Can you work these out from the model? Positions are in its coordinate system, mm. A direction names the side the tool comes from. Coordinates: 2 decimals unless noted, no trailing zeros. Write each loop counter-clockwise with the first axis right and the second up, starting at its lowest first coordinate (ties: lowest second). Pieces come first, ordered by that corner, then holes. Notation, with made-up numbers: (48, 61.5) -> (64, 61.5) arc R35 ccw to (64, 94.5) -> close; hole circle Ø11 at (61, -4). An arc over 180 degrees is marked (long way). Answer as CSV lines item,"result". Start each with the question number.
```python
from build123d import *

# Parameters (mm, degrees)
EXTRUDE_1_DEPTH            = 11.7
EXTRUDE_2_DEPTH            = 20
SKETCH_3_W                 = 3
SKETCH_3_H                 = 2.35
EXTRUDE_3_DEPTH            = 20
EXTRUDE_4_DEPTH            = 28.3
SKETCH_5_W                 = 2.35
SKETCH_5_H                 = 60
EXTRUDE_5_DEPTH            = 14.7
CUT_EXTRUDE_1_REACH        = 70.066
SKETCH_6_W                 = 11
SKETCH_6_H                 = 2.6
CUT_EXTRUDE_2_REACH        = 70.066
CUT_EXTRUDE_3_REACH        = 70.066
HOLE_WIZARD_3_0_3_1_D      = 3
HOLE_WIZARD_3_0_3_1_DEPTH  = 19.132814283
HOLE_WIZARD_3_0_3_2_D      = 3
HOLE_WIZARD_3_0_3_2_DEPTH  = 2.35
HOLE_WIZARD_15_0_15_1_D    = 15
HOLE_WIZARD_3_0_3_3_REACH  = 65.316
HOLE_WIZARD_3_0_3_3_BORE_R = 1.5
HOLE_WIZARD_3_0_3_4_REACH  = 68.474
HOLE_WIZARD_3_0_3_4_BORE_R = 1.5
FILLET_1_R                 = 1
FILLET_2_R                 = 2
FILLET_START               = 2.9999999
FILLET_3_DEPTH             = 3.0000001
FILLET_START_2             = -60
FILLET_3_2_DEPTH           = 60


with BuildPart() as part:
    # Эскиз1 → Бобышка-Вытянуть1 (new body)
    with BuildSketch(Plane(origin=(0, 0, 0), x_dir=(1, 0, 0), z_dir=(0, 1, 0))):
        with BuildLine():
            Line((9, 21.5), (6, 21.5))
            Line((6, 21.5), (6, 8.5))
            Line((6, 8.5), (-10.132814283, 8.5))
            Line((-10.132814283, 8.5), (-8.930469533, -1.11656344))
            ThreePointArc((-8.930469533, -1.11656344), (0.55936312, -8.982600564), (9, 0))
            Line((9, 0), (9, 21.5))
        make_face()
    extrude(amount=-EXTRUDE_1_DEPTH)

    # Эскиз2 → Бобышка-Вытянуть2 (add)
    with BuildSketch(Plane.XZ.offset(11.7)):
        with BuildLine():
            Line((9, -8.5), (-10.132814283, -8.5))
            Line((-10.132814283, -8.5), (-8.930469533, 1.11656344))
            ThreePointArc((-8.930469533, 1.11656344), (0.55936312, 8.982600564), (9, 0))
            Line((9, 0), (9, -8.5))
        make_face()
    extrude(amount=EXTRUDE_2_DEPTH)

    # Эскиз3 → Бобышка-Вытянуть3 (add)
    with BuildSketch(Plane.XZ.offset(11.7)):
        with Locations((7.5, -20.325)):
            Rectangle(SKETCH_3_W, SKETCH_3_H)
    extrude(amount=EXTRUDE_3_DEPTH)

    # Эскиз4 → Бобышка-Вытянуть4 (add)
    with BuildSketch(Plane.XZ.offset(31.7)):
        with BuildLine():
            Line((6, -21.5), (6, -8.5))
            Line((6, -8.5), (-10.132814283, -8.5))
            Line((-10.132814283, -8.5), (-8.930469533, 1.11656344))
            ThreePointArc((-8.930469533, 1.11656344), (0.55936312, 8.982600564), (9, 0))
            Line((9, 0), (9, -21.5))
            Line((9, -21.5), (6, -21.5))
        make_face()
    extrude(amount=EXTRUDE_4_DEPTH)

    # Эскиз5 → Бобышка-Вытянуть5 (add)
    with BuildSketch(Plane.ZY.offset(-6)):
        with Locations((-20.325, -30)):
            Rectangle(SKETCH_5_W, SKETCH_5_H)
    extrude(amount=EXTRUDE_5_DEPTH)

    # Эскиз6 → Вырез-Вытянуть1 (cut, up to next)
    with BuildSketch(Plane(origin=(0, 0, -21.5), x_dir=(-1, 0, 0), z_dir=(0, 0, -1)), mode=Mode.PRIVATE) as cut_extrude_1_sk1:
        with Locations((3.2, -1.3)):
            Rectangle(SKETCH_6_W, SKETCH_6_H)
    cut_extrude_1_tool1 = extrude(cut_extrude_1_sk1.sketch, amount=-CUT_EXTRUDE_1_REACH, mode=Mode.PRIVATE) & part.part
    add(cut_extrude_1_tool1.solids().sort_by_distance((-3.2, -1.3, -21.5))[0], mode=Mode.SUBTRACT)

    # Эскиз7 → Вырез-Вытянуть2 (cut, up to next)
    with BuildSketch(Plane(origin=(0, 0, -21.5), x_dir=(-1, 0, 0), z_dir=(0, 0, -1)), mode=Mode.PRIVATE) as cut_extrude_2_sk1:
        Polygon((8.7, -13.1), (8.7, -6.1), (1.7, -6.1), (1.7, -10.1), (5.7, -10.1), align=None)
    cut_extrude_2_tool1 = extrude(cut_extrude_2_sk1.sketch, amount=-CUT_EXTRUDE_2_REACH, mode=Mode.PRIVATE) & part.part
    add(cut_extrude_2_tool1.solids().sort_by_distance((-5.546154, -8.515385, -21.5))[0], mode=Mode.SUBTRACT)

    # Эскиз8 → Вырез-Вытянуть3 (cut, up to next)
    with BuildSketch(Plane(origin=(0, 0, -21.5), x_dir=(-1, 0, 0), z_dir=(0, 0, -1)), mode=Mode.PRIVATE) as cut_extrude_3_sk1:
        Polygon((8.7, -44.4), (8.7, -36.9), (5.7, -39.9), (1.7, -39.9), (1.7, -41.4), (5.7, -41.4), align=None)
    cut_extrude_3_tool1 = extrude(cut_extrude_3_sk1.sketch, amount=-CUT_EXTRUDE_3_REACH, mode=Mode.PRIVATE) & part.part
    add(cut_extrude_3_tool1.solids().sort_by_distance((-6.353846, -40.65, -21.5))[0], mode=Mode.SUBTRACT)

    # Диаметр отверстия Ø3.0 (3)1
    with Locations(Plane(origin=(9, 0, 0), x_dir=(0, 0, -1), z_dir=(1, 0, 0))):
        with Locations((15, -3.85), (15, -56.15)):
            Hole(HOLE_WIZARD_3_0_3_1_D / 2, depth=HOLE_WIZARD_3_0_3_1_DEPTH)

    # Диаметр отверстия Ø3.0 (3)2
    with Locations(Plane(origin=(0, 0, -21.5), x_dir=(-1, 0, 0), z_dir=(0, 0, -1))):
        with Locations((5.392274393, -21.25)):
            Hole(HOLE_WIZARD_3_0_3_2_D / 2, depth=HOLE_WIZARD_3_0_3_2_DEPTH)

    # Диаметр отверстия Ø15.0 (15)1 (through all)
    with Locations(Plane(origin=(0, 0, 0), x_dir=(1, 0, 0), z_dir=(0, 1, 0))):
        with Locations((0, 0)):
            Hole(HOLE_WIZARD_15_0_15_1_D / 2)

    # Диаметр отверстия Ø3.0 (3)3 bore → Диаметр отверстия Ø3.0 (3)3 (cut, up to next)
    with BuildSketch(Plane(origin=(0, 0, -8.5), x_dir=(-1, 0, 0), z_dir=(0, 0, -1)), mode=Mode.PRIVATE) as hole_wizard_3_0_3_3_sk1:
        with Locations((5.392274393, -21.25)):
            Circle(HOLE_WIZARD_3_0_3_3_BORE_R)
    hole_wizard_3_0_3_3_tool1 = extrude(hole_wizard_3_0_3_3_sk1.sketch, amount=-HOLE_WIZARD_3_0_3_3_REACH, mode=Mode.PRIVATE) & part.part
    add(hole_wizard_3_0_3_3_tool1.solids().sort_by_distance((-5.392274, -21.25, -8.5))[0], mode=Mode.SUBTRACT)

    # Диаметр отверстия Ø3.0 (3)4 bore → Диаметр отверстия Ø3.0 (3)4 (cut, up to next)
    with BuildSketch(Plane.ZY.offset(9.883926163), mode=Mode.PRIVATE) as hole_wizard_3_0_3_4_sk1:
        with Locations((-5.009349323, -13)):
            Circle(HOLE_WIZARD_3_0_3_4_BORE_R)
    hole_wizard_3_0_3_4_tool1 = extrude(hole_wizard_3_0_3_4_sk1.sketch, amount=-HOLE_WIZARD_3_0_3_4_REACH, mode=Mode.PRIVATE) & part.part
    # Диаметр отверстия Ø3.0 (3)4 bore → Диаметр отверстия Ø3.0 (3)4 (cut, up to next)
    with BuildSketch(Plane.ZY.offset(9.883926163), mode=Mode.PRIVATE) as hole_wizard_3_0_3_4_sk2:
        with Locations((-5.009349323, -47)):
            Circle(HOLE_WIZARD_3_0_3_4_BORE_R)
    hole_wizard_3_0_3_4_tool2 = extrude(hole_wizard_3_0_3_4_sk2.sketch, amount=-HOLE_WIZARD_3_0_3_4_REACH, mode=Mode.PRIVATE) & part.part
    add(hole_wizard_3_0_3_4_tool1.solids().sort_by_distance((-9.883926, -13, -5.009349))[0], mode=Mode.SUBTRACT)
    add(hole_wizard_3_0_3_4_tool2.solids().sort_by_distance((-9.883926, -47, -5.009349))[0], mode=Mode.SUBTRACT)

    # Скругление1
    fillet_1_edges = [part.edges().sort_by_distance(p)[0] for p in [
        (-10.132814283, -30, -8.5),
        (6, -45.85, -19.15),
        (6, -5.85, -19.15),
    ]]
    fillet(fillet_1_edges, radius=FILLET_1_R)

    # Скругление2
    fillet_2_edges = [part.edges().sort_by_distance(p)[0] for p in [
        (7, -11.7, -19.15),
        (7.5, -31.7, -8.5),
        (7.5, -11.7, -8.5),
        (7, -31.7, -19.15),
    ]]
    fillet(fillet_2_edges, radius=FILLET_2_R)

    # Скругление3: read off the stored shape, not the designer's step
    # Скругление3 outline → Скругление3 (add)
    with BuildSketch(Plane.YZ.offset(FILLET_START)):
        with BuildLine():
            Line((-13.7, -19.15), (0, -19.15))
            Line((0, -19.15), (0, -8.5))
            Line((0, -8.5), (-13.7, -8.5))
            ThreePointArc((-13.7, -8.5), (-12.285786438, -9.085786438), (-11.7, -10.5))
            Line((-11.7, -10.5), (-11.7, -17.15))
            ThreePointArc((-11.7, -17.15), (-12.285786438, -18.564213562), (-13.7, -19.15))
        make_face()
        with BuildLine():
            Line((-60, -8.5), (-60, -19.15))
            Line((-60, -19.15), (-29.7, -19.15))
            ThreePointArc((-29.7, -19.15), (-31.114213562, -18.564213562), (-31.7, -17.15))
            Line((-31.7, -17.15), (-31.7, -10.5))
            ThreePointArc((-31.7, -10.5), (-31.114213562, -9.085786438), (-29.7, -8.5))
            Line((-29.7, -8.5), (-60, -8.5))
        make_face()
    extrude(amount=FILLET_3_DEPTH)

    # Fillet 3 2 outline → Fillet 3 2 (cut)
    with BuildSketch(Plane(origin=(0, 0, 0), x_dir=(1, 0, 0), z_dir=(0, 1, 0)).offset(FILLET_START_2)):
        with BuildLine():
            ThreePointArc((6, 21.5), (8.121320344, 20.621320344), (9, 18.5))
            Line((9, 18.5), (9, 21.5))
            Line((9, 21.5), (6, 21.5))
        make_face()
        with BuildLine():
            Line((6, 11.5), (6, 18.15))
            ThreePointArc((6, 18.15), (5.707106781, 18.857106781), (5, 19.15))
            Line((5, 19.15), (2.9999999, 19.15))
            Line((2.9999999, 19.15), (3, 8.5))
            ThreePointArc((3, 8.5), (5.121320344, 9.378679656), (6, 11.5))
        make_face()
    extrude(amount=FILLET_3_2_DEPTH, mode=Mode.SUBTRACT)


solid = part.part
```
Q1. For pin 1 (0.7 mm diameter, centred on y = -1.5, z = -20.5, fed in from -X); pin 2 (2 mm diameter, centred on y = -8.5, z = -16, fed in from -X); pin 3 (1.9 mm diameter, centred on x = -4, z = -20.5, fed in from +Y), each with a flat end and sliding along its axis, tell me the tip position at first contact or that it passes through.
Q2. If we mould it in two halves opening along Y, with no side actions, what happens to faces 1 (the face through (-8.7, -52, -20)), 2 (the face through (1.6, 0, -7.5)), 3 (the face through (6.6, -30.9, -8.9))? For each: released by +Y, released by -Y, zero draft, split by the parting line, or undercut.
Q3. I need wall thicknesses on L1, parallel to Z at x = -0.25, y = -5; L2, parallel to Y at x = 7.55, z = -15; L3, parallel to Z at x = 2.5, y = -33. Which ranges of each line are inside material? Lowest first, please.
Q4. Imagine slicing it at A-A (y = -3.85). Write out the boundary of the cut face in (x, z), then the cut area to 3 significant figures.
Q5. Imagine slicing it at D-D (x = -2.75). Write out the boundary of the cut face in (y, z).
Q6. Imagine slicing it at C-C (z = -15.5). Write out the boundary of the cut face in (x, y).
Q7. Which directions (+Z, -Z, +X, -X, +Y, -Y) give clear straight access to the entire face, cutting with the end or side of a thin tool? Please do faces 4 (the face through (7.42, -12.27, -18.55)), 5 (the face through (-6.823, -20.799, -6.383)), 6 (the face through (5.1, -45.06, -9.36)), 7 (the face through (-7.2, -38.4, -20.3)).
Q8. Imagine slicing it at B-B (x = 0). Write out the boundary of the cut face in (y, z), then the cut area to 3 significant figures.
Entries:
1,pin 1,"x = 2.3"
1,pin 2,"x = 6"
1,pin 3,"y = -2.6"
2,face 1,"zero draft"
2,face 2,"released by +Y"
2,face 3,"undercut"
3,L1,"-21.5 to -19.15, -8.5 to -7.5, 7.5 to 9"
3,L2,"-60 to -57.65, -54.65 to -31.7, -11.7 to -5.35, -2.35 to 0"
3,L3,"-21.5 to -19.15, -8.5 to -7.07, 7.07 to 8.65"
4,outline,"(-9.99, -7.38) arc R1 ccw to (-9, -8.5) -> (3, -8.5) arc R3 cw to (6, -11.5) -> (6, -13.5) -> (9, -13.5) -> (9, 0) arc R9 ccw to (-8.93, 1.12) -> close; (-8.7, -21.5) -> (6, -21.5) arc R3 ccw to (9, -18.5) -> (9, -16.5) -> (6, -16.5) -> (6, -18.15) arc R1 cw to (5, -19.15) -> (-8.7, -19.15) -> close; hole circle Ø15 at (0, 0)"
4,area,"173 mm2"
5,outline,"(-60, -21.5) -> (-41.4, -21.5) -> (-41.4, -19.15) -> (-60, -19.15) -> close; (-60, -8.5) -> (0, -8.5) -> (0, -6.98) -> (-60, -6.98) -> close; (-60, 6.98) -> (0, 6.98) -> (0, 8.57) -> (-60, 8.57) -> close; (-39.9, -21.5) -> (-10.1, -21.5) -> (-10.1, -19.15) -> (-39.9, -19.15) -> close; (-6.1, -21.5) -> (-2.6, -21.5) -> (-2.6, -19.15) -> (-6.1, -19.15) -> close"
6,outline,"(6, -60) -> (9, -60) -> (9, -57.56) -> (6, -57.56) -> close; (6, -54.74) -> (9, -54.74) -> (9, -31.7) -> (6, -31.7) -> close; (6, -11.7) -> (9, -11.7) -> (9, -5.26) -> (6, -5.26) -> close; (6, -2.44) -> (9, -2.44) -> (9, 0) -> (6, 0) -> close"
7,face 4,"+X, -X"
7,face 5,"-Z"
7,face 6,"-X, +Y, -Y"
7,face 7,"-Z, -X"
8,outline,"(-60, -21.5) -> (-2.6, -21.5) -> (-2.6, -19.15) -> (-60, -19.15) -> close; (-60, -8.5) -> (0, -8.5) -> (0, -7.5) -> (-60, -7.5) -> close; (-60, 7.5) -> (0, 7.5) -> (0, 9) -> (-60, 9) -> close"
8,area,"285 mm2"
